The figure shows three views and two pictorial views of one solid part (mm, origin at its lowest corner). Answer the questions. A direction names the side the tool comes from. Coordinates: 2 decimals unless noted, no trailing zeros. Write each loop counter-clockwise with the first axis right and the second up, starting at its lowest first coordinate (ties: lowest second). Pieces come first, ordered by that corner, then holes. Notation, with made-up numbers: M 57,-14.5 L 111,-14.5 A17 ccw 111,-4.5 Z; hole C 44.5,49 d9. An arc over 180 degrees is marked long. Write item = value, one per line. Start each with the question number.
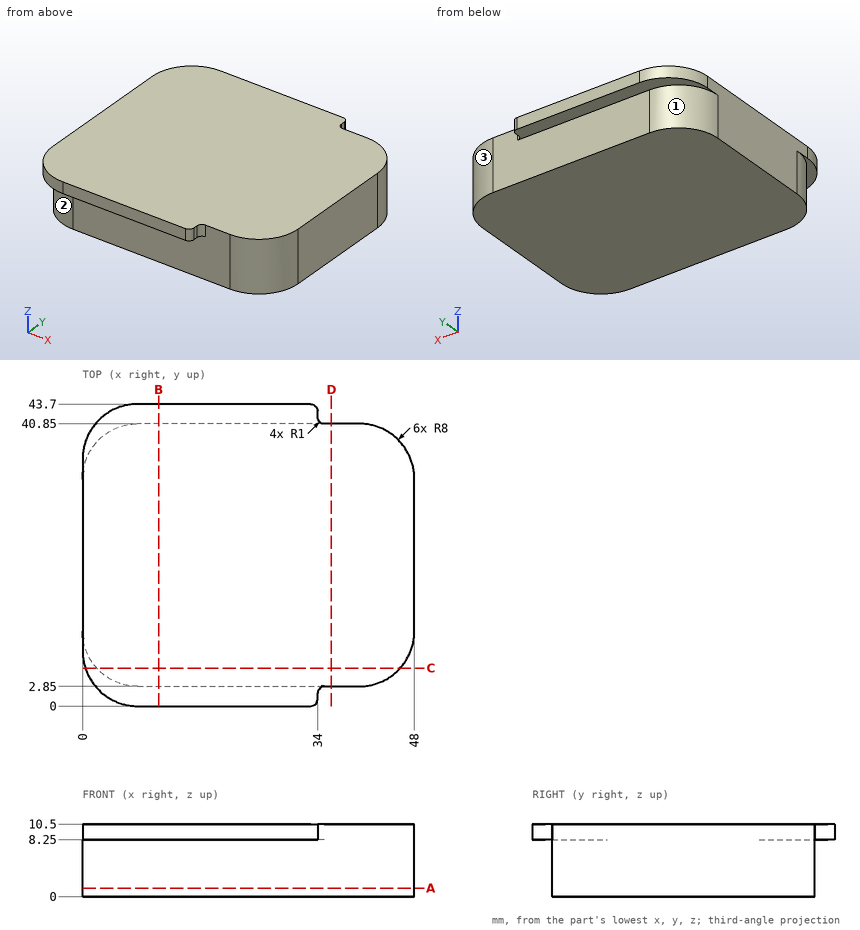
1. The part is cut by section B-B, the plane x = 11. Write down the section's boundary in (y, z), and give its area (3 significant figures).
2. Straight lines are drawn through the part: L1, parallel to Y at x = 9, z = 2.25; L2, parallel to X at y = 39.5, z = 3; L3, parallel to X at y = 38.5, z = 7.75. For each, find the intervals that lie inside material, in ascending order. Write a range as [from, to].
3. The part is cut by section D-D, the plane x = 36. Write down the section's boundary in (y, z).
4. For the marked faces 1, 2 and 3, determine the directions among +Z, -Z, +X, -X, +Y, -Y from which every point of the face is accessible in a straight line to the end or side of a thin tool.
5. Each of these flat-tipped pins is pushed along its axis until it touches: pin 1 (1 mm diameter, centred on x = 34.5, z = 7.5, fed in from -Y); pin 2 (0.7 mm diameter, centred on y = 42.5, z = 10, fed in from +X); pin 3 (3 mm diameter, centred on x = 20.5, z = 3, fed in from +Y). Where does it stop, or does it pass through?
6. The part is cut by section A-A, the plane z = 1.25. Write down the section's boundary in (x, y).
7. The part is cut by section C-C, the plane y = 5.5. Write down the section's boundary in (x, z), and give its area (3 significant figures).
Solution:
q1.outline = M 0,8.25 L 2.85,8.25 L 2.85,0 L 40.85,0 L 40.85,8.25 L 43.7,8.25 L 43.7,10.5 L 0,10.5 Z
q1.area = 412 mm^2
q2.L1 = [2.85, 40.85]
q2.L2 = [3.55, 44.45]
q2.L3 = [2.34, 45.66]
q3.outline = M 2.85,0 L 40.85,0 L 40.85,10.5 L 2.85,10.5 Z
q4.face_1 = -Z, -X, +Y
q4.face_2 = -Z, -X, -Y
q4.face_3 = +Z, -Z, +X, +Y
q5.pin_1 = 2.85
q5.pin_2 = 34
q5.pin_3 = 40.85
q6.outline = M 0,10.85 A8 ccw 8,2.85 L 40,2.85 A8 ccw 48,10.85 L 48,32.85 A8 ccw 40,40.85 L 8,40.85 A8 ccw 0,32.85 Z
q7.outline = M 0.4,8.25 L 2.05,8.25 L 2.05,0 L 45.95,0 L 45.95,10.5 L 0.4,10.5 Z
q7.area = 465 mm^2
